Work out the finished part from the listing and answer in its coordinate system (mm). Face numbers are marked on the shaded views. A direction names the side the tool comes from. Give positions to 0.01 mm unless a question says otherwise; leave off trailing zeros. Write each loop counter-clockwise with the first axis right and the second up, starting at its lowest first coordinate (ties: lowest second). Pieces come first, ordered by that corner, then holes.
1) Given pin 1 Ø8 at (x, z) = (-0.5, 21) entering from +Y; pin 2 Ø1 at (x, y) = (38, 29.5) entering from -Z, each flat-ended and moving along its own axis, determine where each tip first touches the part or whether it passes through.
2) Find section A-A (y = 14). Count the separate pieces of the cut face and the enclosed holes in it, plus the area to 3 significant figures.
3) Find section C-C (x = 9). Determine the outline of the cut face in (y, z).
4) A tool of negligible diameter and unlimited length cuts with its end or side. For the marked faces 1 and 2, from which of +Z, -Z, +X, -X, +Y, -Y can it reach the whole face along a straight path? Write none if from no direction.
5) Determine the mould class of the marked faces 3, 4 and 5 for opening direction Z: pulls with the +Z half, pulls with the -Z half, needs draft (parallel to the pull), parting line crosses it, or undercut.
6) Find section B-B (z = 1.5). Determine the outline of the cut face in (x, y).
7) Straight lines are drawn through the part: probe 1 along X at (y, z) = (10, 33.65) (3 decimals); probe 2 along X at (y, z) = (9, -33). For each, find the intervals that lie inside material, in ascending order.
Autodesk Inventor part; units mm, degrees
ref_plane "YZ Plane" through (0, 0, 0) normal (1, 0, 0) x (0, 1, 0)
ref_plane "XZ Plane" through (0, 0, 0) normal (0, 1, 0) x (-1, 0, 0)
ref_plane "XY Plane" through (0, 0, 0) normal (0, 0, 1) x (1, 0, 0)
sketch "Sketch1" plane through (0, 0, 0) normal (0, 1, 0) x (-1, 0, 0)
  line L0 (-33.65, -40) -> (33.65, -40)
  line L1 (40, -33.65) -> (40, 33.65)
  line L2 (33.65, 40) -> (-33.65, 40)
  line L3 (-40, 33.65) -> (-40, -33.65)
  line L4 (-40, -40) -> (40, 40) construction
  line L5 (40, -40) -> (-40, 40) construction
  arc A0 (40, 33.65) -> (33.65, 40) centre (33.65, 33.65) ccw
  arc A1 (-33.65, 40) -> (-40, 33.65) centre (-33.65, 33.65) ccw
  arc A2 (-40, -33.65) -> (-33.65, -40) centre (-33.65, -33.65) ccw
  arc A3 (33.65, -40) -> (40, -33.65) centre (33.65, -33.65) ccw
  point P0 (0, 0)
  dimension "d0" = 80
  dimension "d1" = 80
  dimension "d2" = 6.35
extrude "Extrusion1" add sketch "Sketch1" along normal blind 25.4
shell "Shell1" thickness 1.7 removed faces 1 at (-11.2167, 25.4, 9.1)
fillet "Fillet1" radius 1.27 8 edges at (-38.1401, 0, -38.1401) (-40, 0, 0) (-38.1401, 0, 38.1401) (0, 0, 40) (38.1401, 0, 38.1401) (40, 0, 0) (38.1401, 0, -38.1401) (0, 0, -40)
sketch "Sketch2" plane through (-33.65, 1.7, 38.3) normal (0, 1, 0) x (1, 0, 0)
  arc A0 (-4.65, 4.65) -> (0, 0) centre (0, 4.65) ccw
  circle A1 centre (0, 4.65) radius 3.175
  circle A2 centre (0, 4.65) radius 1.2
  point P0 (33.65, 38.3)
  dimension "d7" = 6.35
  dimension "d8" = 2.4
extrude "Extrusion2" add sketch "Sketch2" along normal up to surface (23.7 mm away)
mirror "Mirror1" about plane through (0, 0, 0) normal (1, 0, 0) of "Extrusion2"
mirror "Mirror2" about plane through (0, 0, 0) normal (0, 0, 1) of "Extrusion2", "Mirror1"
sketch "Sketch4" plane through (0, 25.4, 0) normal (0, 1, 0) x (1, 0, 0)
  line L0 (-38.3, -33.65) -> (-38.3, 33.65)
  arc A0 (-33.65, 38.3) -> (-38.3, 33.65) centre (-33.65, 33.65) ccw
  line L1 (-33.65, 38.3) -> (33.65, 38.3)
  arc A1 (38.3, 33.65) -> (33.65, 38.3) centre (33.65, 33.65) ccw
  line L2 (38.3, 33.65) -> (38.3, -33.65)
  arc A2 (33.65, -38.3) -> (38.3, -33.65) centre (33.65, -33.65) ccw
  line L3 (33.65, -38.3) -> (-33.65, -38.3)
  arc A3 (-38.3, -33.65) -> (-33.65, -38.3) centre (-33.65, -33.65) ccw
  arc A4 (-40, -33.65) -> (-33.65, -40) centre (-33.65, -33.65) ccw
  line L4 (-33.65, -40) -> (33.65, -40)
  arc A5 (33.65, -40) -> (40, -33.65) centre (33.65, -33.65) ccw
  line L5 (40, -33.65) -> (40, 33.65)
  arc A6 (40, 33.65) -> (33.65, 40) centre (33.65, 33.65) ccw
  line L6 (33.65, 40) -> (-33.65, 40)
  arc A7 (-33.65, 40) -> (-40, 33.65) centre (-33.65, 33.65) ccw
  line L7 (-40, 33.65) -> (-40, -33.65)
  circle A8 centre (-33.65, 33.65) radius 1.2
  circle A9 centre (-33.65, 33.65) radius 3.175
  circle A10 centre (-33.65, -33.65) radius 1.2
  circle A11 centre (-33.65, -33.65) radius 3.175
  circle A12 centre (33.65, -33.65) radius 1.2
  circle A13 centre (33.65, -33.65) radius 3.175
  circle A14 centre (33.65, 33.65) radius 1.2
  circle A15 centre (33.65, 33.65) radius 3.175
  point P0 (0, 0)
extrude "Extrusion4" add sketch "Sketch4" along normal blind 10
sketch "Sketch5" plane through (-33.65, 1.7, 38.3) normal (0, 1, 0) x (1, 0, 0)
  line L0 (71.95, 71.95) -> (71.95, 4.65)
  line L1 (71.95, 13.9457) -> (70.68, 13.9457)
  line L2 (70.68, 13.9457) -> (70.68, 26.6457)
  line L3 (70.68, 26.6457) -> (71.95, 26.6457)
  line L4 (71.95, 26.6457) -> (71.95, 13.9457)
  point P0 (33.65, 38.3)
  dimension "d18" = 1.27
  dimension "d19" = 12.7
extrude "Extrusion5" add sketch "Sketch5" along normal up to surface (33.7 mm away)
sketch "Sketch6" plane through (37.03, 1.7, 11.6543) normal (-1, 0, 0) x (0, 0, 1)
  line L0 (10.75, 30.7) -> (1.75, 30.7)
  line L1 (1.75, 30.7) -> (1.75, 26.7)
  line L2 (1.75, 26.7) -> (10.75, 26.7)
  line L3 (10.75, 26.7) -> (10.75, 30.7)
  line L4 (0, 0) -> (0, 33.7)
  line L5 (21.9957, 33.7) -> (-45.3043, 33.7)
  line L6 (3.05, 17.3) -> (9.45, 17.3)
  line L7 (9.45, 17.3) -> (9.45, 23.7)
  line L8 (9.45, 23.7) -> (3.05, 23.7)
  line L9 (3.05, 23.7) -> (3.05, 17.3)
  line L10 (3.05, 17.3) -> (9.45, 23.7) construction
  line L11 (9.45, 17.3) -> (3.05, 23.7) construction
  point P0 (-11.6543, -1.7)
  point P1 (6.25, 20.5)
  dimension "d22" = 9
  dimension "d23" = 4
  dimension "d24" = 1.75
  dimension "d25" = 3
  dimension "d26" = 6.4
  dimension "d27" = 6.4
  dimension "d28" = 3
extrude "Extrusion6" cut sketch "Sketch6" against normal blind 10
chamfer "Chamfer1" distance 1 angle 45 8 edges at (40, 28.4, 17.9043) (40, 30.4, 22.4043) (40, 32.4, 17.9043) (40, 30.4, 13.4043) (40, 22.2, 21.1043) (40, 22.2, 14.7043) (40, 19, 17.9043) (40, 25.4, 17.9043)
sketch "Sketch7" plane through (40, 1.27, 33.65) normal (1, 0, 0) x (0, 0, -1)
  line L0 (59.68, 14.826) -> (51.806, 14.826)
  line L1 (51.806, 14.826) -> (51.806, 27.78)
  line L2 (51.806, 27.78) -> (59.68, 27.78)
  line L3 (59.68, 27.78) -> (59.68, 14.826)
  line L4 (59.68, 14.826) -> (51.806, 27.78) construction
  line L5 (51.806, 14.826) -> (59.68, 27.78) construction
  line L6 (0, 34.13) -> (67.3, 34.13)
  line L7 (67.3, 0) -> (67.3, 34.13)
  point P0 (33.65, -1.27)
  point P1 (55.743, 21.303)
  dimension "d34" = 7.874
  dimension "d35" = 12.954
  dimension "d36" = 6.35
  dimension "d37" = 7.62
extrude "Extrusion7" cut sketch "Sketch7" against normal blind 25.4
chamfer "Chamfer2" distance 0.762 angle 45 4 edges at (40, 22.573, -18.156) (40, 16.096, -22.093) (40, 29.05, -22.093) (40, 22.573, -26.03)
properties part number "Arduino_case_bottom_JC_Rev2"
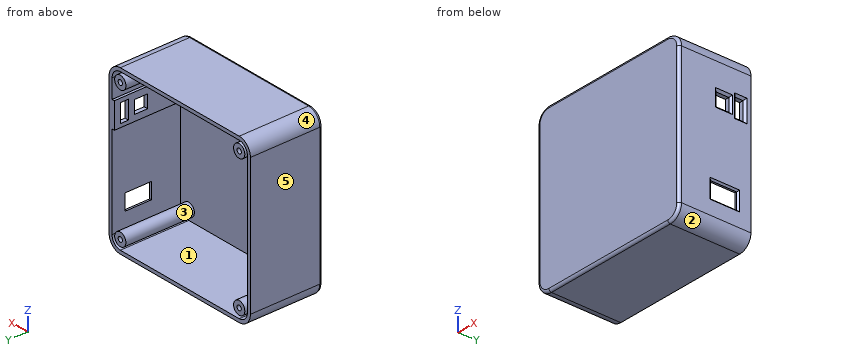
Results:
1. pin 1: stops at y = 1.7
1. pin 2: stops at z = -38.7
2. separate pieces: 5
2. enclosed holes: 5
2. area: 641 mm2
3. outline: (0, -38.73) arc R1.27 ccw to (1.27, -40) - (35.4, -40) - (35.4, -38.3) - (1.7, -38.3) - (1.7, 38.3) - (35.4, 38.3) - (35.4, 40) - (1.27, 40) arc R1.27 ccw to (0, 38.73) - close
4. face 1: +Y
4. face 2: -Z, +X, +Y, -Y
5. face 3: undercut
5. face 4: pulls with the +Z half
5. face 5: needs draft
6. outline: (-40, 1.27) arc R1.27 ccw to (-38.73, 0) - (38.73, 0) arc R1.27 ccw to (40, 1.27) - (40, 35.4) - (38.3, 35.4) - (38.3, 1.7) - (-38.3, 1.7) - (-38.3, 35.4) - (-40, 35.4) - close
7. probe 1: x = -40 to -38.3, -36.825 to -34.85, -32.45 to -30.475, 30.475 to 32.45, 34.85 to 36.825, 38.3 to 40
7. probe 2: x = -40 to -38.3, -36.76 to -34.66, -32.64 to -30.54, 30.54 to 32.64, 34.66 to 36.76, 38.3 to 40
